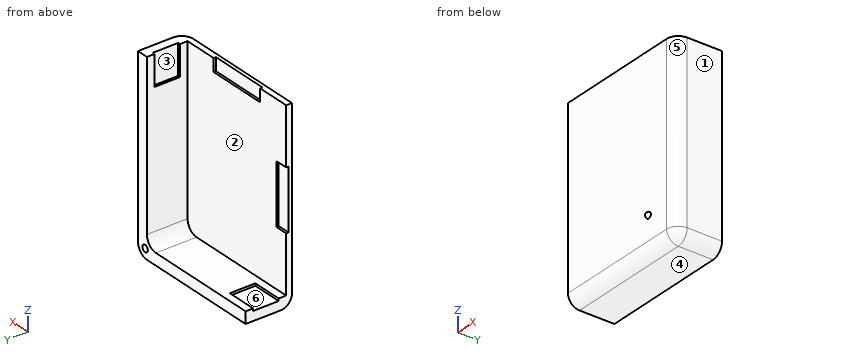
```python
from build123d import *

# Parameters (mm, degrees)
ESQUISSE1_W             = 120
ESQUISSE1_H             = 160
BOSS_EXTRU_1_DEPTH      = 40
CONG_1_R                = 10
CONG_2_R                = 10
ESQUISSE2_W             = 110
ESQUISSE2_H             = 150
ENL_V_MAT_EXTRU_1_DEPTH = 35
CONG_3_R                = 10
ESQUISSE3_R             = 3
ENL_V_MAT_EXTRU_2_DEPTH = 35
ESQUISSE4_R             = 2.5
BOSS_EXTRU_2_DEPTH      = 2.5
CONG_4_R                = 2.5
ESQUISSE5_W             = 11
ESQUISSE5_H             = 52
ESQUISSE5_W_2           = 52
ESQUISSE5_H_2           = 11
ENL_V_MAT_EXTRU_3_DEPTH = 2
ESQUISSE6_W             = 26
ESQUISSE6_H             = 22
ENL_V_MAT_EXTRU_4_DEPTH = 2
ESQUISSE7_W             = 26
ESQUISSE7_H             = 22
ENL_V_MAT_EXTRU_5_DEPTH = 2


with BuildPart() as part:
    # Esquisse1 → Boss.-Extru.1 (new body)
    with BuildSketch(Plane(origin=(0, 0, 0), x_dir=(1, 0, 0), z_dir=(0, 1, 0))):
        with Locations((60, 80)):
            Rectangle(ESQUISSE1_W, ESQUISSE1_H)
    extrude(amount=BOSS_EXTRU_1_DEPTH)

    # Congé1
    cong_1_edges = [part.edges().sort_by_distance(p)[0] for p in [
        (60, 0, -160),
    ]]
    fillet(cong_1_edges, radius=CONG_1_R)

    # Congé2
    cong_2_edges = [part.edges().sort_by_distance(p)[0] for p in [
        (120, 2.928932188, -157.071067812),
        (120, 0, -75),
        (120, 25, -160),
    ]]
    fillet(cong_2_edges, radius=CONG_2_R)

    # Esquisse2 → Enlèv. mat.-Extru.1 (cut)
    with BuildSketch(Plane(origin=(0, 40, 0), x_dir=(1, 0, 0), z_dir=(0, 1, 0))):
        with Locations((55, 75)):
            Rectangle(ESQUISSE2_W, ESQUISSE2_H)
    extrude(amount=-ENL_V_MAT_EXTRU_1_DEPTH, mode=Mode.SUBTRACT)

    # Congé3
    cong_3_edges = [part.edges().sort_by_distance(p)[0] for p in [
        (110, 22.5, -150),
    ]]
    fillet(cong_3_edges, radius=CONG_3_R)

    # Esquisse3 → Enlèv. mat.-Extru.2 (cut)
    with BuildSketch(Plane(origin=(0, 40, 0), x_dir=(1, 0, 0), z_dir=(0, 1, 0))):
        with Locations(Location((112, 152, 0), (0, 0, 270))):
            Circle(ESQUISSE3_R)
    extrude(amount=-ENL_V_MAT_EXTRU_2_DEPTH, mode=Mode.SUBTRACT)

    # Esquisse4 → Boss.-Extru.2 (add)
    with BuildSketch(Plane.XZ):
        with Locations(Location((90, -130, 0), (0, 0, 270))):
            Circle(ESQUISSE4_R)
    extrude(amount=BOSS_EXTRU_2_DEPTH)

    # Congé4
    cong_4_edges = [part.edges().sort_by_distance(p)[0] for p in [
        (90, -2.5, -127.5),
    ]]
    fillet(cong_4_edges, radius=CONG_4_R - 0.0001)  # a hair under: the kernel refuses the full size

    # Esquisse5 → Enlèv. mat.-Extru.3 (cut)
    with BuildSketch(Plane(origin=(0, 5, 0), x_dir=(1, 0, 0), z_dir=(0, 1, 0))):
        with Locations((5.5, 75)):
            Rectangle(ESQUISSE5_W, ESQUISSE5_H)
        with Locations((55, 5.5)):
            Rectangle(ESQUISSE5_W_2, ESQUISSE5_H_2)
    extrude(amount=-ENL_V_MAT_EXTRU_3_DEPTH, mode=Mode.SUBTRACT)

    # Esquisse6 → Enlèv. mat.-Extru.4 (cut)
    with BuildSketch(Plane.XY.offset(-150)):
        with Locations((13, 22.5)):
            Rectangle(ESQUISSE6_W, ESQUISSE6_H)
    extrude(amount=-ENL_V_MAT_EXTRU_4_DEPTH, mode=Mode.SUBTRACT)

    # Esquisse7 → Enlèv. mat.-Extru.5 (cut)
    with BuildSketch(Plane.ZY.offset(-110)):
        with Locations((-13, 22.5)):
            Rectangle(ESQUISSE7_W, ESQUISSE7_H)
    extrude(amount=-ENL_V_MAT_EXTRU_5_DEPTH, mode=Mode.SUBTRACT)


solid = part.part
```
The listing builds one solid part. Answer for the finished solid, in the listing's coordinates (mm). Face numbers are marked on the shaded views. A direction names the side the tool comes from. Give positions to 0.01 mm unless a question says otherwise; leave off trailing zeros. Order: outer loops, then holes, each group sorted by start corner. A loop starts at its lowest first (then second) coordinate and runs counter-clockwise, first axis right, second up. Notation, with made-up numbers: (-25, 79) -> (5, 79) arc R4 cw to (5, 83) -> close; hole circle Ø1 at (86.5, 2). An arc over 180 degrees is marked (long way). Answer as CSV lines item,"result". Start each with the question number.
Q1. Given pin 1 (0.6 mm diameter, centred on y = 4, z = -4, fed in from +X); pin 2 (1.6 mm diameter, centred on x = 49, y = 4, fed in from +Z); pin 3 (1.6 mm diameter, centred on x = 3, y = 3.5, fed in from -Z), each flat-ended and moving along its own axis, determine where each tip first touches the part or whether it passes through.
Q2. A cutting plane is placed at D-D (z = -147). Determine the outline of the cut face in (x, y).
Q3. Determine the mould class of the marked faces 4, 5 and 6 for opening direction Y: pulls with the +Y half, pulls with the -Y half, needs draft (parallel to the pull), parting line crosses it, or undercut.
Q4. A cutting plane is placed at A-A (y = 19). Determine the outline of the cut face in (x, z), then the cut area to 3 significant figures.
Q5. A cutting plane is placed at B-B (z = -42). Determine the outline of the cut face in (x, y), then the cut area to 3 significant figures.
Q6. Which of the six approach directions +Z, -Z, +X, -X, +Y, -Y give full straight-line access (tool end or side, diameter ignored) to the marked faces 1, 2 and 3?
Q7. A cutting plane is placed at C-C (x = 57). Determine the outline of the cut face in (y, z).
Q8. Find the intervals of material crossed by L1, parallel to Y at x = 93.5, z = -143; L2, parallel to Z at x = 53, y = 20; L3, parallel to X at y = 21.5, z = -132, in increasing order.
Results found:
1,pin 1,"x = 118.22"
1,pin 2,"z = -11"
1,pin 3,"z = -158.22"
2,outline,"(0, 0) -> (110, 0) arc R10 ccw to (120, 10) -> (120, 40) -> (107.14, 40) -> (107.14, 5) -> (0, 5) -> close"
3,face 4,"needs draft"
3,face 5,"pulls with the -Y half"
3,face 6,"undercut"
4,outline,"(0, -160) -> (110, -160) arc R10 ccw to (120, -150) -> (120, 0) -> (112, 0) -> (112, -26) -> (110, -26) -> (110, -140) arc R10 cw to (100, -150) -> (26, -150) -> (26, -152) -> (0, -152) -> close; hole circle Ø6 at (112, -152)"
4,area,"2,570 mm2"
5,outline,"(0, 0) -> (110, 0) arc R10 ccw to (120, 10) -> (120, 40) -> (110, 40) -> (110, 5) -> (0, 5) -> close"
5,area,"929 mm2"
6,face 1,"+Z, -Z, +X, +Y, -Y"
6,face 2,"+Z, -X, +Y"
6,face 3,"+Z, -X"
7,outline,"(0, -150) arc R10 ccw to (10, -160) -> (40, -160) -> (40, -150) -> (5, -150) -> (5, -11) -> (3, -11) -> (3, 0) -> (0, 0) -> close"
8,L1,"0 to 5"
8,L2,"-160 to -150"
8,L3,"110 to 120"
